```python
from build123d import *

# Parameters (mm, degrees)
BOSS_EXTRUDE1_DEPTH = 5
CUT_EXTRUDE1_START  = -10
SKETCH3_R           = 2.6
CUT_EXTRUDE1_DEPTH  = 10
FILLET1_R           = 10
FILLET2_R           = 3
SKETCH4_R           = 2.6
CUT_EXTRUDE2_DEPTH  = 10
CUT_EXTRUDE3_DEPTH  = 4
CUT_EXTRUDE4_DEPTH  = 10


with BuildPart() as part:
    # Sketch1 → Boss-Extrude1 (new body)
    with BuildSketch(Plane.XY):
        with BuildLine():
            Line((-42.619167718, 65.881324086), (73.380832282, 65.881324086))
            ThreePointArc((73.380832282, 65.881324086), (75.502152626, 65.002644429), (76.380832282, 62.881324086))
            Line((76.380832282, 62.881324086), (76.380832282, -41.118675914))
            ThreePointArc((76.380832282, -41.118675914), (75.502152626, -43.239996258), (73.380832282, -44.118675914))
            Line((73.380832282, -44.118675914), (-42.619167718, -44.118675914))
            ThreePointArc((-42.619167718, -44.118675914), (-44.740488061, -43.239996258), (-45.619167718, -41.118675914))
            Line((-45.619167718, -41.118675914), (-45.619167718, 62.881324086))
            ThreePointArc((-45.619167718, 62.881324086), (-44.740488061, 65.002644429), (-42.619167718, 65.881324086))
        make_face()
    extrude(amount=BOSS_EXTRUDE1_DEPTH)

    # Sketch3 → Cut-Extrude1 (cut)
    with BuildSketch(Plane.XY.offset(5).offset(CUT_EXTRUDE1_START)):
        with BuildLine():
            Line((-42.619167718, 65.881324086), (6.780832282, 65.881324086))
            Line((6.780832282, 65.881324086), (6.780832282, 81.136513461))
            Line((6.780832282, 81.136513461), (-45.619167718, 81.136513461))
            Line((-45.619167718, 81.136513461), (-45.619167718, 62.881324086))
            ThreePointArc((-45.619167718, 62.881324086), (-44.740488061, 65.002644429), (-42.619167718, 65.881324086))
        make_face()
        with BuildLine():
            Line((-2.217047099, 54.63427273), (6.780832282, 65.881324086))
            Line((6.780832282, 65.881324086), (-42.619167718, 65.881324086))
            ThreePointArc((-42.619167718, 65.881324086), (-44.740488061, 65.002644429), (-45.619167718, 62.881324086))
            Line((-45.619167718, 62.881324086), (-45.619167718, 50.881324086))
            Line((-45.619167718, 50.881324086), (-10.025654488, 50.881324086))
            ThreePointArc((-10.025654488, 50.881324086), (-5.693825403, 51.868263741), (-2.217047099, 54.63427273))
        make_face()
        with BuildLine():
            ThreePointArc((73.380832282, 65.881324086), (75.502152626, 65.002644429), (76.380832282, 62.881324086))
            Line((76.380832282, 62.881324086), (76.380832282, 81.136513461))
            Line((76.380832282, 81.136513461), (23.980832282, 81.136513461))
            Line((23.980832282, 81.136513461), (23.980832282, 65.881324086))
            Line((23.980832282, 65.881324086), (73.380832282, 65.881324086))
        make_face()
        with BuildLine():
            ThreePointArc((32.978711664, 54.63427273), (36.455489968, 51.868263741), (40.787319053, 50.881324086))
            Line((40.787319053, 50.881324086), (76.380832282, 50.881324086))
            Line((76.380832282, 50.881324086), (76.380832282, 62.881324086))
            ThreePointArc((76.380832282, 62.881324086), (75.502152626, 65.002644429), (73.380832282, 65.881324086))
            Line((73.380832282, 65.881324086), (23.980832282, 65.881324086))
            Line((23.980832282, 65.881324086), (32.978711664, 54.63427273))
        make_face()
        with BuildLine():
            Line((76.380832282, -41.118675914), (76.380832282, -29.118675914))
            Line((76.380832282, -29.118675914), (40.787319053, -29.118675914))
            ThreePointArc((40.787319053, -29.118675914), (36.455489968, -30.105615569), (32.978711664, -32.871624558))
            Line((32.978711664, -32.871624558), (23.980832282, -44.118675914))
            Line((23.980832282, -44.118675914), (73.380832282, -44.118675914))
            ThreePointArc((73.380832282, -44.118675914), (75.502152626, -43.239996258), (76.380832282, -41.118675914))
        make_face()
        with BuildLine():
            Line((76.380832282, -59.373865289), (76.380832282, -41.118675914))
            ThreePointArc((76.380832282, -41.118675914), (75.502152626, -43.239996258), (73.380832282, -44.118675914))
            Line((73.380832282, -44.118675914), (23.980832282, -44.118675914))
            Line((23.980832282, -44.118675914), (23.980832282, -59.373865289))
            Line((23.980832282, -59.373865289), (76.380832282, -59.373865289))
        make_face()
        with BuildLine():
            Line((-42.619167718, -44.118675914), (6.780832282, -44.118675914))
            Line((6.780832282, -44.118675914), (-2.217047099, -32.871624558))
            ThreePointArc((-2.217047099, -32.871624558), (-5.693825403, -30.105615569), (-10.025654488, -29.118675914))
            Line((-10.025654488, -29.118675914), (-45.619167718, -29.118675914))
            Line((-45.619167718, -29.118675914), (-45.619167718, -41.118675914))
            ThreePointArc((-45.619167718, -41.118675914), (-44.740488061, -43.239996258), (-42.619167718, -44.118675914))
        make_face()
        with BuildLine():
            Line((6.780832282, -59.373865289), (6.780832282, -44.118675914))
            Line((6.780832282, -44.118675914), (-42.619167718, -44.118675914))
            ThreePointArc((-42.619167718, -44.118675914), (-44.740488061, -43.239996258), (-45.619167718, -41.118675914))
            Line((-45.619167718, -41.118675914), (-45.619167718, -59.373865289))
            Line((-45.619167718, -59.373865289), (6.780832282, -59.373865289))
        make_face()
        with Locations((15.380832282, -31.118675914)):
            Circle(SKETCH3_R)
    extrude(amount=CUT_EXTRUDE1_DEPTH, mode=Mode.SUBTRACT)

    # Fillet1
    fillet1_edges = [part.edges().sort_by_distance(p)[0] for p in [
        (6.780832282, 65.881324086, 2.5),
        (23.980832282, 65.881324086, 2.5),
        (23.980832282, -44.118675914, 2.5),
        (6.780832282, -44.118675914, 2.5),
    ]]
    fillet(fillet1_edges, radius=FILLET1_R)

    # Fillet2
    fillet2_edges = [part.edges().sort_by_distance(p)[0] for p in [
        (-45.619167718, -29.118675914, 2.5),
        (-45.619167718, 50.881324086, 2.5),
        (76.380832282, 50.881324086, 2.5),
        (76.380832282, -29.118675914, 2.5),
    ]]
    fillet(fillet2_edges, radius=FILLET2_R)

    # Sketch4 → Cut-Extrude2 (cut)
    with BuildSketch(Plane.XY.offset(5)):
        with Locations((15.380832282, 52.881324086)):
            Circle(SKETCH4_R)
    extrude(amount=-CUT_EXTRUDE2_DEPTH, mode=Mode.SUBTRACT)

    # Sketch5 → Cut-Extrude3 (cut)
    with BuildSketch(Plane.XY.offset(5)):
        with BuildLine():
            Line((-30.619167718, 40.881324086), (61.380832282, 40.881324086))
            ThreePointArc((61.380832282, 40.881324086), (64.916366188, 39.416857992), (66.380832282, 35.881324086))
            Line((66.380832282, 35.881324086), (66.380832282, -14.118675914))
            ThreePointArc((66.380832282, -14.118675914), (64.916366188, -17.65420982), (61.380832282, -19.118675914))
            Line((61.380832282, -19.118675914), (-30.619167718, -19.118675914))
            ThreePointArc((-30.619167718, -19.118675914), (-34.154701623, -17.65420982), (-35.619167718, -14.118675914))
            Line((-35.619167718, -14.118675914), (-35.619167718, 35.881324086))
            ThreePointArc((-35.619167718, 35.881324086), (-34.154701623, 39.416857992), (-30.619167718, 40.881324086))
        make_face()
    extrude(amount=-CUT_EXTRUDE3_DEPTH, mode=Mode.SUBTRACT)

    # Sketch6 → Cut-Extrude4 (cut)
    with BuildSketch(Plane.XY.offset(5)):
        with BuildLine():
            Line((23.165898511, 60.881324086), (7.595766054, 60.881324086))
            ThreePointArc((7.595766054, 60.881324086), (3.25131348, 59.888306479), (-0.230315515, 57.106470452))
            Line((-0.230315515, 57.106470452), (-2.058004159, 58.560279644))
            Line((-2.058004159, 58.560279644), (6.679710473, 70.400464375))
            Line((6.679710473, 70.400464375), (28.478804217, 70.400464375))
            Line((28.478804217, 70.400464375), (32.819668724, 58.560279644))
            Line((32.819668724, 58.560279644), (30.99198008, 57.106470452))
            ThreePointArc((30.99198008, 57.106470452), (27.510351085, 59.888306479), (23.165898511, 60.881324086))
        make_face()
        with BuildLine():
            Line((28.478804217, -48.637816204), (32.819668724, -36.797631473))
            Line((32.819668724, -36.797631473), (30.99198008, -35.343822281))
            ThreePointArc((30.99198008, -35.343822281), (27.510351085, -38.125658307), (23.165898511, -39.118675914))
            Line((23.165898511, -39.118675914), (7.595766054, -39.118675914))
            ThreePointArc((7.595766054, -39.118675914), (3.25131348, -38.125658307), (-0.230315515, -35.343822281))
            Line((-0.230315515, -35.343822281), (-2.058004159, -36.797631473))
            Line((-2.058004159, -36.797631473), (6.679710473, -48.637816204))
            Line((6.679710473, -48.637816204), (28.478804217, -48.637816204))
        make_face()
    extrude(amount=-CUT_EXTRUDE4_DEPTH, mode=Mode.SUBTRACT)


solid = part.part
```
Verification items for the finished model (mm, model axes). A direction names the side the tool comes from. Coordinates: 2 decimals unless noted, no trailing zeros. Order: outer loops, then holes, each group sorted by start corner. A loop starts at its lowest first (then second) coordinate and runs counter-clockwise, first axis right, second up. Notation, with made-up numbers: (60.25, 9) -> (77.25, 9) arc R32 cw to (77.25, 40) -> close; hole circle Ø10 at (38, -8). An arc over 180 degrees is marked (long way). Put each result on its own line as item: value. Start each with the question number.
1) Cross-section at B-B (x = 20). Enter the section's corners in (y, z), plus the area to 3 significant figures.
2) Go/stop test with flat-tipped pins: pin 1 (1.5 mm diameter, centred on x = -23.5, z = 3.5, fed in from +Y); pin 2 (2 mm diameter, centred on x = 34.5, z = 1.5, fed in from -Y); pin 3 (2 mm diameter, centred on x = 37, z = 2.5, fed in from +Y). Record where each tip stops, or that it passes through.
3) Cross-section at A-A (y = 5.5). Enter the section's corners in (x, z).
4) Cross-section at C-C (z = 1.75). State how many separate pieces and enclosed holes the cut face has, plus the area to 3 significant figures.
5) Tool access check on faces 1 (the flat face through (-1.21, -34.13, 2.46)), 2 (the flat face through (-27, 50.881, 2)), 3 (the cylindrical face through (75.479, 50.026, 2.535)), 4 (the cylindrical face through (-34.19, 39.38, 3.03)), 5 (the flat face through (57, -29.119, 2)). Record the directions out of +Z, -Z, +X, -X, +Y, -Y that give a thin tool (end or side, any length) a straight path to the whole face; none if there is none.
6) Release check for a two-part mould opening along X. For faces 6 (the flat face through (16, 45, 5)), 7 (the flat face through (-45.619, 10, 2)), 8 (the flat face through (16, -19.119, 3)) record: pulls with the +X half, pulls with the -X half, needs draft (parallel to the pull), parting line crosses it, or undercut.
7) Material ranges on L1, parallel to Y at x = -11, z = 2.4; L2, parallel to X at y = 13, z = 3.65; L3, parallel to Y at x = -34.5, z = 0.55, recorded low to high.
Geometry check:
1. outline: (-39.12, 0) -> (60.88, 0) -> (60.88, 5) -> (40.88, 5) -> (40.88, 1) -> (-19.12, 1) -> (-19.12, 5) -> (-39.12, 5) -> close
1. area: 260 mm^2
2. pin 1: stops at y = 50.88
2. pin 2: stops at y = -32.27
2. pin 3: stops at y = 52.1
3. outline: (-45.62, 0) -> (76.38, 0) -> (76.38, 5) -> (66.38, 5) -> (66.38, 1) -> (-35.62, 1) -> (-35.62, 5) -> (-45.62, 5) -> close
4. separate pieces: 1
4. enclosed holes: 3
4. area: 4,280 mm^2
5. face 1: +Z, -Z, -X, -Y
5. face 2: +Z, -Z, -X, +Y
5. face 3: +Z, -Z, +X, +Y
5. face 4: +Z
5. face 5: +Z, -Z, +X, -Y
6. face 6: needs draft
6. face 7: pulls with the -X half
6. face 8: undercut
7. L1: y = -29.12 to -19.12, 40.88 to 50.88
7. L2: x = -45.62 to -35.62, 66.38 to 76.38
7. L3: y = -29.12 to 50.88
